Can you work these out from the drawing? Everything is in mm from the part's minimum corner. A direction names the side the tool comes from. Round coordinates to 2 decimals unless told otherwise and drop trailing zeros. Loops run counter-clockwise (first coordinate to the right, second up) from the corner with the lowest first, then second, coordinate; pieces in that order, holes last. Notation, with made-up numbers: M 26.25,89.5 L 30.25,89.5 A12 ccw 30.25,110.5 Z; hole C 71,-38 d9. An arc over 180 degrees is marked long. Use a Markdown table: item, result.
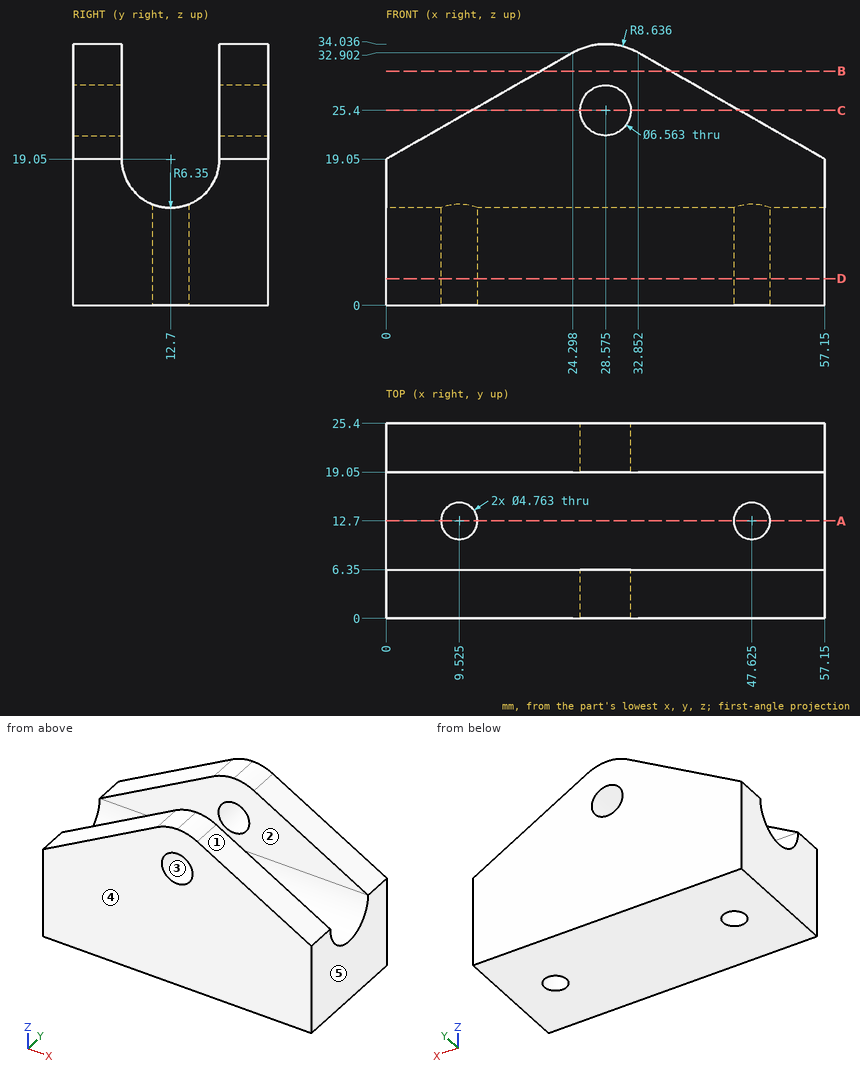
Q1. Imagine slicing it at C-C, the plane z = 25.4. Please give me the cut outline in (x, y).
Return value:
| item | result |
|---|---|
| outline | M 11.14,0 L 25.29,0 L 25.29,6.35 L 11.14,6.35 Z; M 11.14,19.05 L 25.29,19.05 L 25.29,25.4 L 11.14,25.4 Z; M 31.86,0 L 46.01,0 L 46.01,6.35 L 31.86,6.35 Z; M 31.86,19.05 L 46.01,19.05 L 46.01,25.4 L 31.86,25.4 Z |
Q2. Imagine slicing it at A-A, the plane y = 12.7. Please give me the cut outline in (x, z).
Return value:
| item | result |
|---|---|
| outline | M 0,0 L 7.14,0 L 7.14,12.7 L 0,12.7 Z; M 11.91,0 L 45.24,0 L 45.24,12.7 L 11.91,12.7 Z; M 50.01,0 L 57.15,0 L 57.15,12.7 L 50.01,12.7 Z |
Q3. For the marked faces 1 and 2, which set-ups out of +Z, -Z, +X, -X, +Y, -Y let a thin tool reach every point of the face, with its end or its side?
Return value:
| item | result |
|---|---|
| face 1 | +Z, +X, +Y, -Y |
| face 2 | +Z, +X, -X |
Q4. Will these pins go through, and if not, where does the flat tip stop? P1, Ø4, axis at x = 19.5, y = 15.5, coming from the +Z side (1 decimal); P2, Ø4.5, axis at x = 47.625, y = 12.7, coming from the +Z side; P3, Ø7.5, axis at x = 33, z = 23.5, coming from the -Y side; P4, Ø10, axis at y = 9.5, z = 30.5, coming from the +X side (1 decimal).
Return value:
| item | result |
|---|---|
| P1 | stops at z = 14.9 |
| P2 | passes through |
| P3 | stops at y = 0 |
| P4 | stops at x = 43.9 |
Q5. Imagine slicing it at B-B, the plane z = 30.5. Please give me the cut outline in (x, y).
Return value:
| item | result |
|---|---|
| outline | M 20.08,0 L 37.07,0 L 37.07,6.35 L 20.08,6.35 Z; M 20.08,19.05 L 37.07,19.05 L 37.07,25.4 L 20.08,25.4 Z |
Q6. I need wall thicknesses on line 1 (X direction, y = 12.7, z = 8.75); line 2 (Y direction, x = 49, z = 19). Which ranges of each line are inside material? Lowest first, please. Write a range as from..to.
Return value:
| item | result |
|---|---|
| line 1 | x = 0..7.14, 11.91..45.24, 50.01..57.15 |
| line 2 | y = 0..6.35, 19.05..25.4 |
Q7. Imagine slicing it at D-D, the plane z = 3.5. Give the number of separate pieces and of enclosed holes in the cut face, then the cut area to 3 significant figures.
Return value:
| item | result |
|---|---|
| separate pieces | 1 |
| enclosed holes | 2 |
| area | 1,420 mm^2 |
Q8. We'd pull the mould along X, two halves only. Please class the marked faces 3, 4 and 5: pulls with the +X half, pulls with the -X half, needs draft (parallel to the pull), parting line crosses it, or undercut.
Return value:
| item | result |
|---|---|
| face 3 | undercut |
| face 4 | needs draft |
| face 5 | pulls with the +X half |
